```python
from build123d import *

# Parameters (mm, degrees)
SKETCH4_W           = 24.633837396
SKETCH4_H           = 19.082768461
SKETCH4_W_2         = 5
SKETCH4_H_2         = 5
MAINBRACKET_DEPTH   = 3.5
SKETCH3_R           = 2
BOSS_EXTRUDE2_DEPTH = 13
SKETCH6_R           = 1.5
BOSS_EXTRUDE3_DEPTH = 5
SKETCH7_R           = 2.125
CUT_EXTRUDE1_DEPTH  = 1


with BuildPart() as part:
    # Sketch4 → MainBracket (new body)
    with BuildSketch(Plane(origin=(0, 0, 0), x_dir=(1, 0, 0), z_dir=(0, 1, 0))):
        Polygon((-25.001052975, 23.597895529), (25.52718448, 23.597895529), (27.52718448, 21.597895529), (27.52718448, 18.397895529), (25.52718448, 16.397895529), (15.338231538, 16.397895529), (15.338231538, -31.590979949), (12.338231538, -34.590979949), (-1.661768462, -34.590979949), (-4.661768462, -31.590979949), (-4.661768462, -15.921260677), (-16.583029139, -4), (-16.583029139, 16.421906692), (-25.001052975, 16.421906692), (-27.001052975, 18.421906692), (-27.001052975, 21.597895529), align=None)
        with Locations((0.008956485, 13.000441896)):
            Rectangle(SKETCH4_W, SKETCH4_H, mode=Mode.SUBTRACT)
        with Locations((-0.204070078, -11.047717724)):
            Rectangle(SKETCH4_W_2, SKETCH4_H_2, mode=Mode.SUBTRACT)
    extrude(amount=MAINBRACKET_DEPTH)

    # Sketch3 → Boss-Extrude2 (add)
    with BuildSketch(Plane(origin=(0, 0, 0), x_dir=(1, 0, 0), z_dir=(0, 1, 0))):
        with Locations(Location((-24.011269627, 19.663273311, 0), (0, 0, 270))):
            Circle(SKETCH3_R)
        with Locations(Location((24.107482847, 18.27469294, 0), (0, 0, 270))):
            Circle(SKETCH3_R)
        with Locations(Location((8.917908931, -32.088026328, 0), (0, 0, 270))):
            Circle(SKETCH3_R)
    extrude(amount=-BOSS_EXTRUDE2_DEPTH)

    # Sketch6 → Boss-Extrude3 (add)
    with BuildSketch(Plane.XZ.offset(13)):
        with Locations(Location((-24.011269627, -19.663273311, 0), (0, 0, 270))):
            Circle(SKETCH6_R)
        with Locations(Location((8.917908931, 32.088026328, 0), (0, 0, 270))):
            Circle(SKETCH6_R)
        with Locations(Location((24.107482847, -18.27469294, 0), (0, 0, 270))):
            Circle(SKETCH6_R)
    extrude(amount=BOSS_EXTRUDE3_DEPTH)

    # Sketch7 → Cut-Extrude1 (cut)
    with BuildSketch(Plane(origin=(0, 3.5, 0), x_dir=(1, 0, 0), z_dir=(0, 1, 0))):
        with Locations(Location((-0.204070078, -21.047717724, 0), (0, 0, 270))):
            Circle(SKETCH7_R)
        with Locations(Location((-0.204070078, -4.047717724, 0), (0, 0, 270))):
            Circle(SKETCH7_R)
        with Locations(Location((9.795929922, -11.047717724, 0), (0, 0, 270))):
            Circle(SKETCH7_R)
    extrude(amount=-CUT_EXTRUDE1_DEPTH, mode=Mode.SUBTRACT)


solid = part.part
```
Geometry: final body of the model. Coordinates: model frame, mm. A direction names the side the tool comes from. Coordinates: 2 decimals unless noted, no trailing zeros. Order: outer loops, then holes, each group sorted by start corner. A loop starts at its lowest first (then second) coordinate and runs counter-clockwise, first axis right, second up. Notation, with made-up numbers: M 1.5,30 L 53.5,30 A18 ccw 53.5,39 Z; hole C 39.5,41.25 d10. An arc over 180 degrees is marked long. Answer as CSV lines item,"result".
Q1. Section A-A on x = 3. Return the cut outline in (y, z).
Answers:
outline,"M 0,-23.6 L 3.5,-23.6 L 3.5,-22.54 L 0,-22.54 Z; M 0,-3.46 L 3.5,-3.46 L 3.5,34.59 L 0,34.59 Z"
Q2. Line query: probe 1 along Z at (x, y) = (10, 0.5); probe 2 along Y at (x, z) = (15, -17); probe 3 along X at (y, z) = (2, 20.5). Output: solid intervals per line, ascending. Write a range as [from, to].
Answers:
probe 1,"z = [-23.6, -22.54], [-3.46, 34.59]"
probe 2,"y = [0, 3.5]"
probe 3,"x = [-4.66, 15.34]"
Q3. Section B-B on z = -14. Return the cut outline in (x, y), and give its area (3 significant figures).
Answers:
outline,"M -16.58,0 L -12.31,0 L -12.31,3.5 L -16.58,3.5 Z; M 12.33,0 L 15.34,0 L 15.34,3.5 L 12.33,3.5 Z"
area,"25.5 mm^2"
Q4. Set-up query: faces 1 (the flat face through (0, 2, 8.548)), 2 (the cylindrical face through (-22.028, -6.409, -19.924)), 3 (the flat face through (0, 2.5, 4)). Return all of +Z, -Z, +X, -X, +Y, -Y with unobstructed straight access to the full face (end or side cutting, diameter ignored); none if empty.
Answers:
face 1,"+Y, -Y"
face 2,"-Y"
face 3,"+Y"
Q5. Draft query along Z for faces 4 (the flat face through (0, 2, -22.542)), 5 (the flat face through (0, 2, -3.459)), 6 (the flat face through (-24, -18, -20)), 7 (the flat face through (-25.99, 1.73, -17.41)). Return one class per face: pulls with the +Z half, pulls with the -Z half, needs draft (parallel to the pull), parting line crosses it, or undercut.
Answers:
face 4,"undercut"
face 5,"undercut"
face 6,"needs draft"
face 7,"pulls with the +Z half"
Q6. First-contact query: P1, Ø3, axis at y = 1.5, z = -12.5, coming from the -X side; P2, Ø12, axis at x = 1, z = 11, coming from the -Y side; P3, Ø3, axis at y = 0, z = -16.5, coming from the -X side; P4, Ø8, axis at x = 1, y = -9.5, coming from the +Z side. Flat tips, straight axial feed; report the tip coordinate or a pass-through.
Answers:
P1,"stops at x = -16.58"
P2,"stops at y = 0"
P3,"stops at x = -26.58"
P4,"passes through"
Q7. Section C-C on y = -14. Return the cut outline in (x, z), and give its area (3 significant figures).
Answers:
outline,"C -24.01,-19.66 d3; C 8.92,32.09 d3; C 24.11,-18.27 d3"
area,"21.2 mm^2"
Q8. Section D-D on z = -2.5. Return the cut outline in (x, y), and give its area (3 significant figures).
Answers:
outline,"M -16.58,0 L 15.34,0 L 15.34,3.5 L -16.58,3.5 Z"
area,"112 mm^2"
